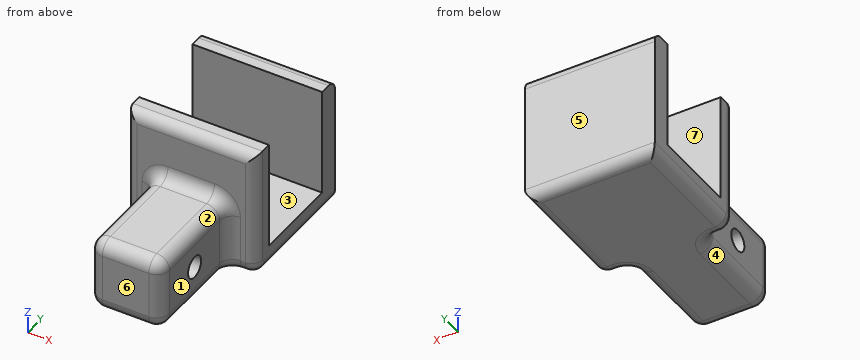
```python
from build123d import *

# Parameters (mm, degrees)
F0_W      = 30
F0_H      = 30
F1_DEPTH  = 5
F2_W      = 30
F2_H      = 4.9
F3_DEPTH  = 25
F4_W      = 16.75
F4_H      = 16.75
F5_DEPTH  = 25
F6_R      = 3
F7_R      = 2.5
F9_R      = 2.5
F10_DEPTH = 16.75


# Not quite as in the source:
# - two fillets or chamfers of one size are made in one step
# - a feature names something its author has since deleted; it is built from what else it names


with BuildPart() as f1:
    # F0 (on Top) → F1 (new body)
    with BuildSketch(Plane.XY):
        with Locations((15, 15)):
            Rectangle(F0_W, F0_H)
    extrude(amount=F1_DEPTH)

    # F2 (on face) → F3 (join)
    with BuildSketch(Plane.XY.offset(5)):
        with Locations((15, 27.55)):
            Rectangle(F2_W, F2_H)
        with Locations((15, 2.45)):
            Rectangle(F2_W, F2_H)
    extrude(amount=F3_DEPTH)

    # F4 (on face) → F5 (join)
    with BuildSketch(Plane.XZ):
        with Locations((15, 8.375)):
            Rectangle(F4_W, F4_H)
    extrude(amount=F5_DEPTH)

    # F6
    f6_edges = [f1.edges().sort_by_distance(p)[0] for p in [
        (6.625, -25, 8.375),
        (23.375, 0, 8.375),
        (23.375, -12.5, 0),
        (23.375, -12.5, 16.75),
        (23.375, -25, 8.375),
        (3.3125, 0, 0),
        (6.625, 0, 8.375),
        (15, 0, 16.75),
        (26.6875, 0, 0),
        (6.625, -12.5, 0),
        (15, -25, 0),
        (6.625, -12.5, 16.75),
        (15, -25, 16.75),
    ]]
    fillet(f6_edges, radius=F6_R)

    # F7
    f7_edges = [f1.edges().sort_by_distance(p)[0] for p in [
        (15, 30, 30),
        (15, 0, 30),
        (15, 30, 0),
        (30, 16.5, 0),
        (0, 16.5, 0),
        (0, 0, 16.5),
        (0, 0.87868, 0.87868),
        (30, 0, 16.5),
        (30, 0.87868, 0.87868),
    ]]
    fillet(f7_edges, radius=F7_R)

    # F9 (on face) → F10 (cut, through all)
    with BuildSketch(Plane.YZ.offset(23.375)):
        with Locations((-12.5, 8.375)):
            Circle(F9_R)
    extrude(amount=-F10_DEPTH, mode=Mode.SUBTRACT)


solid = f1.part
```
Verification items for the finished model (mm, model axes). Face numbers are marked on the shaded views. A direction names the side the tool comes from. Give positions to 0.01 mm unless a question says otherwise; leave off trailing zeros. Loops run counter-clockwise (first coordinate to the right, second up) from the corner with the lowest first, then second, coordinate; pieces in that order, holes last.
1. Section check C-C, the plane y = -5. Enter the section's corners in (x, z) (3 decimals).
2. Set-up check for the marked faces 1, 2, 3 and 4: record each of +Z, -Z, +X, -X, +Y, -Y from which the full face is reachable in a straight line by a thin tool's end or side.
3. Thickness scan on line 1 (Y direction, x = 17, z = 8.5); line 2 (Z direction, x = 13, y = -12.5) (3 decimals); line 3 (Y direction, x = 25.5, z = 19.75). Record the ranges inside material, lowest first.
4. Mould release check, pull along Y, two halves, no side actions. Record for the marked faces 5, 6 and 7: released by +Y, released by -Y, zero draft, split by the parting line, or undercut.
5. Section check B-B, the plane z = 26.5. Enter the section's corners in (x, y), then the cut area to 3 significant figures.
6. Section check A-A, the plane y = -12.5. Enter the section's corners in (x, z) (3 decimals), then the cut area to 3 significant figures.
7. Section check D-D, the plane x = 16.5. Enter the section's corners in (y, z) (3 decimals), then the cut area to 3 significant figures.
8. Go/stop test with flat-tipped pins: pin 1 Ø6 at (x, y) = (14, 14) entering from +Z; pin 2 Ø6 at (y, z) = (-17.5, 4) entering from +X (3 decimals); pin 3 Ø5.5 at (y, z) = (-14.5, 8) entering from -X (3 decimals); pin 4 Ø1.5 at (y, z) = (13, 5.5) entering from +X. Record where each tip stops, or that it passes through.
Geometry says:
1. outline: (6.625, 3) arc R3 ccw to (9.625, 0) - (20.375, 0) arc R3 ccw to (23.375, 3) - (23.375, 13.75) arc R3 ccw to (20.375, 16.75) - (9.625, 16.75) arc R3 ccw to (6.625, 13.75) - close
2. face 1: +Z, -Z, +X, -Y
2. face 2: +Z, +X, -Y
2. face 3: +Z, +X, -X
2. face 4: -Z, -X, -Y
3. line 1: y = -25 to -15, -10 to 4.9, 25.1 to 30
3. line 2: z = 0 to 5.875, 10.875 to 16.75
3. line 3: y = 0 to 4.9, 25.1 to 30
4. face 5: released by +Y
4. face 6: released by -Y
4. face 7: undercut
5. outline: (0, 2.5) arc R2.5 ccw to (2.5, 0) - (27.5, 0) arc R2.5 ccw to (30, 2.5) - (30, 4.9) - (0, 4.9) - close; (0, 25.1) - (30, 25.1) - (30, 30) - (0, 30) - close
5. area: 291 mm2
6. outline: (6.625, 3) arc R3 ccw to (9.625, 0) - (20.375, 0) arc R3 ccw to (23.375, 3) - (23.375, 5.875) - (6.625, 5.875) - close; (6.625, 10.875) - (23.375, 10.875) - (23.375, 13.75) arc R3 ccw to (20.375, 16.75) - (9.625, 16.75) arc R3 ccw to (6.625, 13.75) - close
6. area: 189 mm2
7. outline: (-25, 3) arc R3 ccw to (-22, 0) - (27.5, 0) arc R2.5 ccw to (30, 2.5) - (30, 27.5) arc R2.5 ccw to (27.5, 30) - (25.1, 30) - (25.1, 5) - (4.9, 5) - (4.9, 30) - (2.5, 30) arc R2.5 ccw to (0, 27.5) - (0, 19.75) arc R3 cw to (-3, 16.75) - (-22, 16.75) arc R3 ccw to (-25, 13.75) - close; hole circle Ø5 at (-12.5, 8.375)
7. area: 788 mm2
8. pin 1: stops at z = 5
8. pin 2: stops at x = 23.375
8. pin 3: stops at x = 6.625
8. pin 4: stops at x = 30
